```python
from build123d import *

# Parameters (mm, degrees)
SKETCH_1_W           = 7.62
SKETCH_1_H           = 3.96
EXTRUDE_1_DEPTH      = 10
CUT_EXTRUDE_1_DEPTH  = 8.5
EXTRUDE_2_DEPTH      = 4
EXTRUDE_2_DEPTH_BACK = 9
SKETCH_3_W           = 1
SKETCH_3_H           = 1


with BuildPart() as part:
    # 草图1 → 拉伸1 (new body)
    with BuildSketch(Plane(origin=(0, 0, 0), x_dir=(1, 0, 0), z_dir=(0, 1, 0))):
        Rectangle(SKETCH_1_W, SKETCH_1_H)
    extrude(amount=EXTRUDE_1_DEPTH)

    # 草图2 → 切除-拉伸1 (cut)
    with BuildSketch(Plane(origin=(0, 10, 0), x_dir=(-1, 0, 0), z_dir=(0, 1, 0))):
        with BuildLine():
            Line((-2.81, 1.144818304), (-2.81, 1.98))
            Line((-2.81, 1.98), (3.06, 1.98))
            Line((3.06, 1.98), (3.06, -1.98))
            Line((3.06, -1.98), (-2.81, -1.98))
            Line((-2.81, -1.98), (-2.81, -1.144818304))
            ThreePointArc((-2.81, -1.144818304), (-3.31, 0), (-2.81, 1.144818304))
        make_face()
    extrude(amount=-CUT_EXTRUDE_1_DEPTH, mode=Mode.SUBTRACT)

    # 草图3 → 拉伸2 (add, two sides: drawn at the far end of the back side and taken through both)
    with BuildSketch(Plane.XZ.offset(-EXTRUDE_2_DEPTH_BACK)):
        with Locations((-0.31, 0)):
            Rectangle(SKETCH_3_W, SKETCH_3_H)
    extrude(amount=EXTRUDE_2_DEPTH + EXTRUDE_2_DEPTH_BACK)


solid = part.part
```
The model under review builds one solid part; all positions refer to its coordinate system, in mm. A direction names the side the tool comes from. Round coordinates to 2 decimals unless told otherwise and drop trailing zeros. Loops run counter-clockwise (first coordinate to the right, second up) from the corner with the lowest first, then second, coordinate; pieces in that order, holes last. Notation, with made-up numbers: (84.25, 41.25) - (115.25, 41.25) arc R28 cw to (115.25, 66.25) - close; hole circle Ø7 at (31, 70.25). An arc over 180 degrees is marked (long way). Use a Markdown table: item, result. Add a question column.
Q1. Machinability: for faces 5 (the face through (0, 5, -0.5)), 6 (the face through (0, 9, 0)), 7 (the face through (3.31, 5.81, -0.02)), 8 (the face through (0, -2, -0.5)), 9 (the face through (0, -2, 0.5)), which of the approach directions +Z, -Z, +X, -X, +Y, -Y give a long, thin tool a straight path to every point of the face, cutting with its end or side? Answer none if there is none.
Q2. For probe 1 along X at (y, z) = (2.25, 0.1); probe 2 along X at (y, z) = (3, 1.6); probe 3 along X at (y, z) = (7.75, -0.45), list the stretches that pass through material, from the lowest coordinate up.
Q3. Add section A-A (y = 8.5). State the section outline as (x, z) points, plus the area to 3 significant figures.
Q4. Add section B-B (z = -1.3). State the section outline as (x, y) points.
Q5. Insertion check: pin 1 Ø3 at (x, y) = (2, 8) entering from -Z; pin 2 Ø0.5 at (x, y) = (-0.5, 4.5) entering from -Z; pin 3 Ø1.1 at (y, z) = (-2.5, 0) entering from -X; pin 4 Ø0.5 at (y, z) = (-2, 0) entering from +X. Each pin has a flat end and moves straight along its axis. Give the tip position at first contact, or say it passes through.
Q6. Add section C-C (x = 2). State the section outline as (y, z) points.
Q7. Add section D-D (y = -3). State the section outline as (x, z) points.
Q8. The part is to be moulded in two halves that separate along X. For faces 1 (the face through (-0.81, -2, 0)), 2 (the face through (0, 1, -1.98)), 3 (the face through (0.19, 5, 0)), 4 (the face through (0.19, -2, 0)), say which applies: pulls with the +X half, pulls with the -X half, needs draft (parallel to the pull), parting line crosses it, or undercut.
Worked answers:
| question | item | result |
|---|---|---|
| 1 | face 5 | -Z, +Y |
| 1 | face 6 | +Z, -Z, +Y |
| 1 | face 7 | +Y |
| 1 | face 8 | -Z, +X, -X, -Y |
| 1 | face 9 | +Z, +X, -X, -Y |
| 2 | probe 1 | -3.81 to -3.06, -0.81 to 0.19, 3.31 to 3.81 |
| 2 | probe 2 | -3.81 to -3.06, 2.81 to 3.81 |
| 2 | probe 3 | -3.81 to -3.06, -0.81 to 0.19, 3.24 to 3.81 |
| 3 | outline | (-3.81, -1.98) - (-3.06, -1.98) - (-3.06, 1.98) - (-3.81, 1.98) - close; (-0.81, -0.5) - (0.19, -0.5) - (0.19, 0.5) - (-0.81, 0.5) - close; (2.81, -1.98) - (3.81, -1.98) - (3.81, 1.98) - (2.81, 1.98) - (2.81, 1.14) arc R1.56 cw to (2.81, -1.14) - close |
| 3 | area | 7.14 mm² |
| 4 | outline | (-3.81, 0) - (3.81, 0) - (3.81, 10) - (2.81, 10) - (2.81, 1.5) - (-3.06, 1.5) - (-3.06, 10) - (-3.81, 10) - close |
| 5 | pin 1 | z = -1.98 |
| 5 | pin 2 | z = -0.5 |
| 5 | pin 3 | x = -0.81 |
| 5 | pin 4 | x = 0.19 |
| 6 | outline | (0, -1.98) - (1.5, -1.98) - (1.5, 1.98) - (0, 1.98) - close |
| 7 | outline | (-0.81, -0.5) - (0.19, -0.5) - (0.19, 0.5) - (-0.81, 0.5) - close |
| 8 | face 1 | pulls with the -X half |
| 8 | face 2 | needs draft |
| 8 | face 3 | undercut |
| 8 | face 4 | pulls with the +X half |
